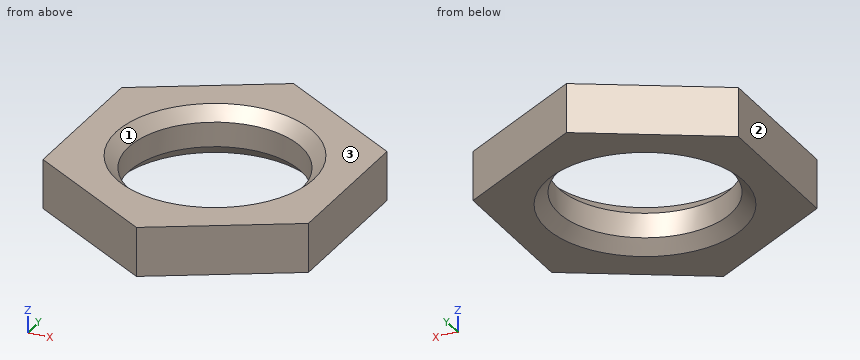
from build123d import *

# Parameters (mm, degrees)
SKETCH019_R             = 3.5
PAD011_DEPTH            = 2
CHAMFER004_SIZE         = 0.5
CHAMFER005_SIZE         = 0.5
BODY007_PITCH_ANGLE     = 90
BODY007_PLACEMENT_ANGLE = 90


with BuildPart() as part:
    # Sketch019 → Pad011 (new body)
    with BuildSketch(Plane.YZ):
        Polygon((5.375, -3.103258), (5.375, 3.103258), (0, 6.206515), (-5.375, 3.103258), (-5.375, -3.103258), (0, -6.206515), align=None)
        Circle(SKETCH019_R, mode=Mode.SUBTRACT)
    extrude(amount=PAD011_DEPTH)

    # Chamfer004
    chamfer004_edges = [part.edges().sort_by_distance(p)[0] for p in [
        (0, -3.5, 0),
    ]]
    chamfer(chamfer004_edges, length=CHAMFER004_SIZE)

    # Chamfer005
    chamfer005_edges = [part.edges().sort_by_distance(p)[0] for p in [
        (2, -3.5, 0),
    ]]
    chamfer(chamfer005_edges, length=CHAMFER005_SIZE)


with BuildPart() as part_1:
    # Body007 pitch: moved
    add(part.part.rotate(Axis((0, 0, 0), (0, 1, 0)), BODY007_PITCH_ANGLE))


with BuildPart() as part_2:
    # Body007 placement: moved
    add(part_1.part.moved(Location((0, 0, -3.1))).rotate(Axis((0, 0, -3.1), (0, 0, 1)), BODY007_PLACEMENT_ANGLE))


solid = part_2.part
Check sheet for the modelled part. Datum: model origin and axes. Units: mm. Face numbers are marked on the shaded views. Give positions to 0.01 mm unless a question says otherwise; leave off trailing zeros. Write each loop counter-clockwise with the first axis right and the second up, starting at its lowest first coordinate (ties: lowest second). Pieces come first, ordered by that corner, then holes. Notation, with made-up numbers: (-29.5, 21) -> (-11.5, 21) arc R22 cw to (-11.5, 56) -> close; hole circle Ø9 at (22, 19.5). An arc over 180 degrees is marked (long way). Write item = value, one per line.
Item 1: Release check for a two-part mould opening along X. For the marked faces 1, 2 and 3 record: +X half, -X half, draft (parallel to the pull), parting line (faces both ways), or undercut.
Output:
face_1 = undercut
face_2 = -X half
face_3 = draft
Item 2: Sectioned sample at A-A on y = 0. Record the boundary of the cut face in (x, z) (3 decimals).
Output:
outline = (-5.375, -5.1) -> (-4, -5.1) -> (-3.5, -4.6) -> (-3.5, -3.6) -> (-4, -3.1) -> (-5.375, -3.1) -> close; (3.5, -4.6) -> (4, -5.1) -> (5.375, -5.1) -> (5.375, -3.1) -> (4, -3.1) -> (3.5, -3.6) -> close
Item 3: Scan lines: probe 1 along X at (y, z) = (-0.5, -4.9) (3 decimals); probe 2 along Y at (x, z) = (-3, -4.2); probe 3 along Y at (x, z) = (2, -3.55). Record each from-to range of solid material in increasing order. Write a range as from..to.
Output:
probe_1 = -5.375..-3.767, 3.767..5.375
probe_2 = -4.47..-1.8, 1.8..4.47
probe_3 = -5.05..-2.93, 2.93..5.05
Item 4: Sectioned sample at C-C on x = 4.75. Record the boundary of the cut face in (y, z).
Output:
outline = (-3.46, -5.1) -> (3.46, -5.1) -> (3.46, -3.1) -> (-3.46, -3.1) -> close
Item 5: Gauge pin test, flat end, axial feed: pin 1 (3 mm diameter, centred on x = -1, y = -2, fed in from +Z). Record the tip position at first contact, or that the pin passes through.
Output:
pin_1 = -3.36
Item 6: Sectioned sample at B-B on z = -3.85. Record the boundary of the cut face in (x, y) (3 decimals), and give its area (3 significant figures).
Output:
outline = (-5.375, -3.103) -> (0, -6.207) -> (5.375, -3.103) -> (5.375, 3.103) -> (0, 6.207) -> (-5.375, 3.103) -> close; hole circle Ø7 at (0, 0)
area = 61.6 mm^2
Item 7: Sectioned sample at D-D on y = 5.25. Record the boundary of the cut face in (x, z).
Output:
outline = (-1.66, -5.1) -> (1.66, -5.1) -> (1.66, -3.1) -> (-1.66, -3.1) -> close
